Geometry check sheet. Reference: the model listing, model coordinates, mm. A direction names the side the tool comes from. Round coordinates to 2 decimals unless told otherwise and drop trailing zeros. Order: outer loops, then holes, each group sorted by start corner. A loop starts at its lowest first (then second) coordinate and runs counter-clockwise, first axis right, second up.
(1) Sectioned sample at A-A (y = -1.75). Record the boundary of the cut face in (x, z).
(2) Set-up check for faces 1 (the face through (3, 0, 1.2)), 2 (the face through (0.058, 5.097, 4.148)), 3 (the face through (2.66, 0, 4)), 4 (the face through (-2.66, 0, 4)): record each of +Z, -Z, +X, -X, +Y, -Y from which the full face is reachable in a straight line by a thin tool's end or side.
(3) Sectioned sample at C-C (z = 0.5). Record the boundary of the cut face in (x, y), plus the area to 3 significant figures.
(4) Go/stop test with flat-tipped pins: pin 1 (1 mm diameter, centred on x = -2, z = 4.5, fed in from +Y); pin 2 (4 mm diameter, centred on x = -1, y = 0, fed in from -Z); pin 3 (4 mm diameter, centred on x = -2.5, z = 5.5, fed in from -Y); pin 4 (4 mm diameter, centred on y = 0, z = 3.5, fed in from -X). Record where each tip stops, or that it passes through.
(5) Sectioned sample at D-D (z = 6.5). Record the boundary of the cut face in (x, y).
(6) Material ranges on line 1 along Z through (x, y) = (-2, 4.75); line 2 along X through (y, z) = (1, 2.5); line 3 along X through (y, z) = (3.5, 0.5), recorded low to high.
(7) Sectioned sample at B-B (x = 0). Record the boundary of the cut face in (y, z), plus the area to 3 significant figures.
from build123d import *

# Parameters (mm, degrees)
BOSS_EXTRUDE1_DEPTH = 1.2
BOSS_EXTRUDE2_DEPTH = 6.48
FILLET1_R           = 0.5


with BuildPart() as part:
    # Sketch1 → Boss-Extrude1 (new body)
    with BuildSketch(Plane.XY):
        with BuildLine():
            Line((-3.8, -2.43766), (-3.8, 2.43766))
            ThreePointArc((-3.8, 2.43766), (0, 6.23766), (3.8, 2.43766))
            Line((3.8, 2.43766), (3.8, -2.43766))
            ThreePointArc((3.8, -2.43766), (0, -6.23766), (-3.8, -2.43766))
        make_face()
    extrude(amount=BOSS_EXTRUDE1_DEPTH)

    # Sketch2 → Boss-Extrude2 (add)
    with BuildSketch(Plane.XY.offset(1.2)):
        with BuildLine():
            Line((2.66, -2.43766), (2.66, 2.43766))
            ThreePointArc((2.66, 2.43766), (0, 5.09766), (-2.66, 2.43766))
            Line((-2.66, 2.43766), (-2.66, -2.43766))
            ThreePointArc((-2.66, -2.43766), (0, -5.09766), (2.66, -2.43766))
        make_face()
    extrude(amount=BOSS_EXTRUDE2_DEPTH)

    # Fillet1
    fillet1_edges = [part.edges().sort_by_distance(p)[0] for p in [
        (0, -5.09766, 7.68),
        (2.66, 0, 7.68),
        (0, 5.09766, 7.68),
        (-2.66, 0, 7.68),
    ]]
    fillet(fillet1_edges, radius=FILLET1_R)


solid = part.part
Answer below:
1. outline: (-3.8, 0) - (3.8, 0) - (3.8, 1.2) - (2.66, 1.2) - (2.66, 7.18) arc R0.5 ccw to (2.16, 7.68) - (-2.16, 7.68) arc R0.5 ccw to (-2.66, 7.18) - (-2.66, 1.2) - (-3.8, 1.2) - close
2. face 1: +Z
2. face 2: +Z, +Y
2. face 3: +Z, +X, +Y, -Y
2. face 4: +Z, -X, +Y, -Y
3. outline: (-3.8, -2.44) arc R3.8 ccw to (3.8, -2.44) - (3.8, 2.44) arc R3.8 ccw to (-3.8, 2.44) - close
3. area: 82.4 mm2
4. pin 1: stops at y = 4.63
4. pin 2: stops at z = 0
4. pin 3: stops at y = -5.05
4. pin 4: stops at x = -2.66
5. outline: (-2.66, -2.44) arc R2.66 ccw to (2.66, -2.44) - (2.66, 2.44) arc R2.66 ccw to (-2.66, 2.44) - close
6. line 1: z = 0 to 1.2
6. line 2: x = -2.66 to 2.66
6. line 3: x = -3.65 to 3.65
7. outline: (-6.24, 0) - (6.24, 0) - (6.24, 1.2) - (5.1, 1.2) - (5.1, 7.18) arc R0.5 ccw to (4.6, 7.68) - (-4.6, 7.68) arc R0.5 ccw to (-5.1, 7.18) - (-5.1, 1.2) - (-6.24, 1.2) - close
7. area: 80.9 mm2
